Can you work these out from the drawing? Everything is in mm from the part's minimum corner. Coordinates: 2 decimals unless noted, no trailing zeros. Order: outer loops, then holes, each group sorted by start corner. A loop starts at its lowest first (then second) coordinate and runs counter-clockwise, first axis right, second up. Notation, with made-up numbers: (0, 88.25) -> (8, 88.25) arc R30 cw to (8, 116.25) -> close; hole circle Ø8 at (-16.5, 86). An arc over 180 degrees is marked (long way). Answer in a Markdown table with one row per item.
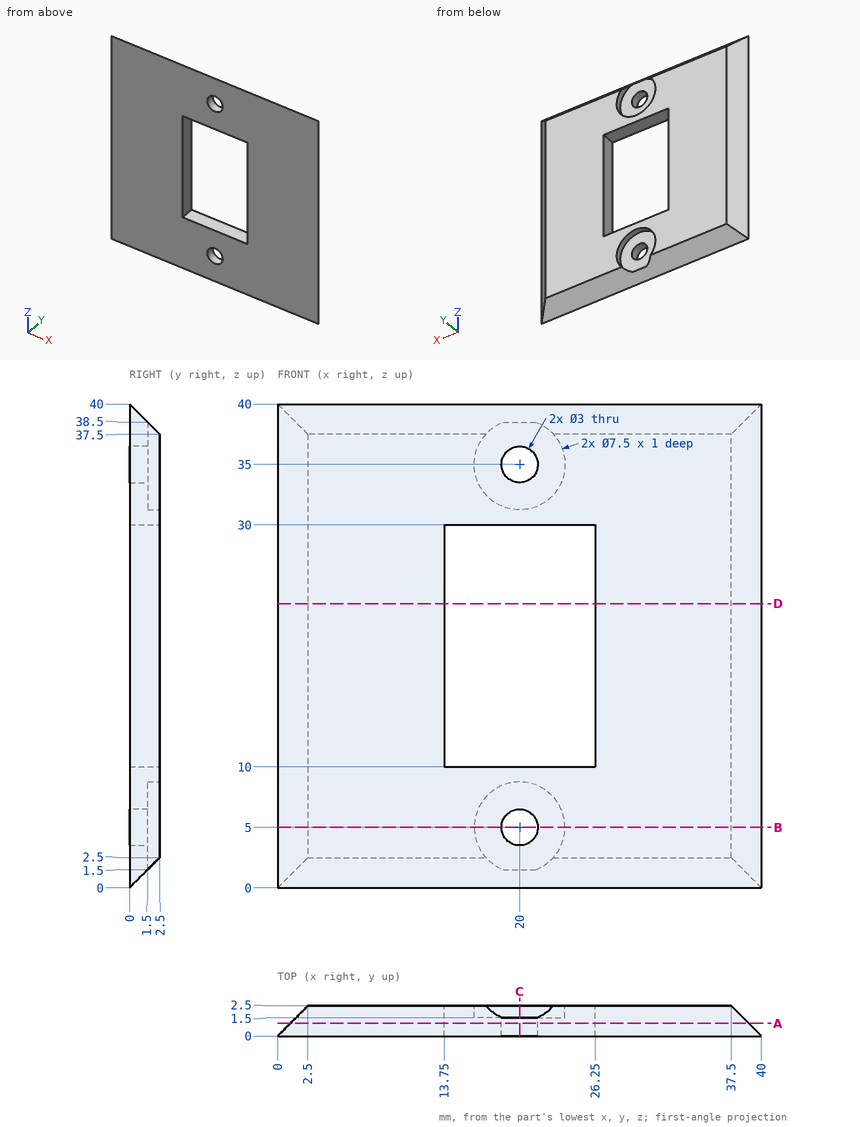
(1) I need wall thicknesses on line 1 (Z direction, x = 20, y = 2.2); line 2 (Z direction, x = 26, y = 0.9); line 3 (X direction, y = 2.05, z = 20). Which ranges of each line are inside material? Lowest first, please. Write a range as [from, to].
Response values:
| item | result |
|---|---|
| line 1 | [8.75, 10], [30, 31.25] |
| line 2 | [0.9, 10], [30, 39.1] |
| line 3 | [2.05, 13.75], [26.25, 37.95] |
(2) Suppose I cut it at B-B (z = 5). Please give me the cut outline in (x, y), and give its area (4 significant figures).
Response values:
| item | result |
|---|---|
| outline | (0, 0) -> (18.5, 0) -> (18.5, 1.5) -> (16.25, 1.5) -> (16.25, 2.5) -> (2.5, 2.5) -> close; (21.5, 0) -> (40, 0) -> (37.5, 2.5) -> (23.75, 2.5) -> (23.75, 1.5) -> (21.5, 1.5) -> close |
| area | 81.75 mm2 |
(3) Suppose I cut it at D-D (z = 23.5). Please give me the cut outline in (x, y).
Response values:
| item | result |
|---|---|
| outline | (0, 0) -> (13.75, 0) -> (13.75, 2.5) -> (2.5, 2.5) -> close; (26.25, 0) -> (40, 0) -> (37.5, 2.5) -> (26.25, 2.5) -> close |
(4) Will these pins go through, and if not, where does the flat tip stop? pin 1 Ø0.8 at (y, z) = (1.5, 17) entering from -X; pin 2 Ø1.2 at (x, y) = (22, 1) entering from +Z; pin 3 Ø1 at (x, y) = (31.5, 2) entering from +Z.
Response values:
| item | result |
|---|---|
| pin 1 | x = 1.1 |
| pin 2 | z = 39.6 |
| pin 3 | z = 38.5 |
(5) Suppose I cut it at A-A (y = 1.05). Please give me the cut outline in (x, z), and give its area (3 significant figures).
Response values:
| item | result |
|---|---|
| outline | (1.05, 1.05) -> (38.95, 1.05) -> (38.95, 38.95) -> (1.05, 38.95) -> close; hole (13.75, 10) -> (26.25, 10) -> (26.25, 30) -> (13.75, 30) -> close; hole circle Ø3 at (20, 5); hole circle Ø3 at (20, 35) |
| area | 1,170 mm2 |
(6) Suppose I cut it at C-C (x = 20). Please give me the cut outline in (y, z), and give its area (4 significant figures).
Response values:
| item | result |
|---|---|
| outline | (0, 0) -> (1.5, 1.5) -> (1.5, 3.5) -> (0, 3.5) -> close; (0, 6.5) -> (1.5, 6.5) -> (1.5, 8.75) -> (2.5, 8.75) -> (2.5, 10) -> (0, 10) -> close; (0, 30) -> (2.5, 30) -> (2.5, 31.25) -> (1.5, 31.25) -> (1.5, 33.5) -> (0, 33.5) -> close; (0, 36.5) -> (1.5, 36.5) -> (1.5, 38.5) -> (0, 40) -> close |
| area | 21.25 mm2 |
